Can you work these out from the model? Positions are in its coordinate system, mm. Coordinates: 2 decimals unless noted, no trailing zeros. Loops run counter-clockwise (first coordinate to the right, second up) from the corner with the lowest first, then second, coordinate; pieces in that order, holes last.
```python
from build123d import *

# Parameters (mm, degrees)
SKETCH1_R           = 88.9
BOSS_EXTRUDE1_DEPTH = 3.175
CUT_EXTRUDE3_DEPTH  = 1.5875
SKETCH3_R           = 14.224
CUT_EXTRUDE4_DEPTH  = 4.175
CUT_EXTRUDE5_DEPTH  = 4.175


with BuildPart() as part:
    # Sketch1 → Boss-Extrude1 (new body)
    with BuildSketch(Plane.XY):
        Circle(SKETCH1_R)
    extrude(amount=BOSS_EXTRUDE1_DEPTH)

    # Sketch2 → Cut-Extrude3 (cut)
    with BuildSketch(Plane(origin=(0, 0, 0), x_dir=(-1, 0, 0), z_dir=(0, 0, -1))):
        with BuildLine():
            ThreePointArc((-77.771132281, -43.068097053), (-76.989658396, -44.45), (-76.183632281, -45.81772771))
            Line((-76.183632281, -45.81772771), (-1.5875, -2.749630657))
            Line((-1.5875, -2.749630657), (-1.5875, -41.700369343))
            ThreePointArc((-1.5875, -41.700369343), (0, -41.275), (1.5875, -41.700369343))
            Line((1.5875, -41.700369343), (1.5875, -2.749630657))
            Line((1.5875, -2.749630657), (76.183632281, -45.81772771))
            ThreePointArc((76.183632281, -45.81772771), (76.989658396, -44.45), (77.771132281, -43.068097053))
            Line((77.771132281, -43.068097053), (3.175, 0))
            Line((3.175, 0), (36.907329198, 19.475369343))
            ThreePointArc((36.907329198, 19.475369343), (35.745198541, 20.6375), (35.319829198, 22.225))
            Line((35.319829198, 22.225), (1.5875, 2.749630657))
            Line((1.5875, 2.749630657), (1.5875, 88.885824763))
            ThreePointArc((1.5875, 88.885824763), (0, 88.9), (-1.5875, 88.885824763))
            Line((-1.5875, 88.885824763), (-1.5875, 2.749630657))
            Line((-1.5875, 2.749630657), (-35.319829198, 22.225))
            ThreePointArc((-35.319829198, 22.225), (-35.745198541, 20.6375), (-36.907329198, 19.475369343))
            Line((-36.907329198, 19.475369343), (-3.175, 0))
            Line((-3.175, 0), (-77.771132281, -43.068097053))
        make_face()
    extrude(amount=-CUT_EXTRUDE3_DEPTH, mode=Mode.SUBTRACT)

    # Sketch3 → Cut-Extrude4 (cut, through all)
    with BuildSketch(Plane.XY.offset(3.175)):
        Circle(SKETCH3_R)
    extrude(amount=-CUT_EXTRUDE4_DEPTH, mode=Mode.SUBTRACT)

    # Sketch2_4 → Cut-Extrude5 (cut, through all)
    with BuildSketch(Plane(origin=(0, 0, 0), x_dir=(-1, 0, 0), z_dir=(0, 0, -1))):
        with BuildLine():
            Line((-41.669829198, 22.225), (-36.907329198, 19.475369343))
            ThreePointArc((-36.907329198, 19.475369343), (-35.745198541, 20.6375), (-35.319829198, 22.225))
            Line((-35.319829198, 22.225), (-40.082329198, 24.974630657))
            ThreePointArc((-40.082329198, 24.974630657), (-41.244459855, 23.8125), (-41.669829198, 22.225))
        make_face()
        with BuildLine():
            ThreePointArc((-41.669829198, 22.225), (-40.082329198, 19.475369343), (-36.907329198, 19.475369343))
            Line((-36.907329198, 19.475369343), (-41.669829198, 22.225))
        make_face()
        with BuildLine():
            Line((-40.082329198, 24.974630657), (-35.319829198, 22.225))
            ThreePointArc((-35.319829198, 22.225), (-36.907329198, 24.974630657), (-40.082329198, 24.974630657))
        make_face()
        with BuildLine():
            ThreePointArc((35.319829198, 22.225), (35.745198541, 20.6375), (36.907329198, 19.475369343))
            Line((36.907329198, 19.475369343), (41.669829198, 22.225))
            ThreePointArc((41.669829198, 22.225), (41.244459855, 23.8125), (40.082329198, 24.974630657))
            Line((40.082329198, 24.974630657), (35.319829198, 22.225))
        make_face()
        with BuildLine():
            ThreePointArc((40.082329198, 24.974630657), (36.907329198, 24.974630657), (35.319829198, 22.225))
            Line((35.319829198, 22.225), (40.082329198, 24.974630657))
        make_face()
        with BuildLine():
            Line((41.669829198, 22.225), (36.907329198, 19.475369343))
            ThreePointArc((36.907329198, 19.475369343), (40.082329198, 19.475369343), (41.669829198, 22.225))
        make_face()
        with BuildLine():
            Line((-1.5875, -47.199630657), (-1.5875, -41.700369343))
            ThreePointArc((-1.5875, -41.700369343), (-3.175, -44.45), (-1.5875, -47.199630657))
        make_face()
        with BuildLine():
            ThreePointArc((1.5875, -41.700369343), (0, -41.275), (-1.5875, -41.700369343))
            Line((-1.5875, -41.700369343), (-1.5875, -47.199630657))
            ThreePointArc((-1.5875, -47.199630657), (0, -47.625), (1.5875, -47.199630657))
            Line((1.5875, -47.199630657), (1.5875, -41.700369343))
        make_face()
        with BuildLine():
            ThreePointArc((3.175, -44.45), (2.749630657, -42.8625), (1.5875, -41.700369343))
            Line((1.5875, -41.700369343), (1.5875, -47.199630657))
            ThreePointArc((1.5875, -47.199630657), (2.749630657, -46.0375), (3.175, -44.45))
        make_face()
    extrude(amount=-CUT_EXTRUDE5_DEPTH, mode=Mode.SUBTRACT)


solid = part.part
```
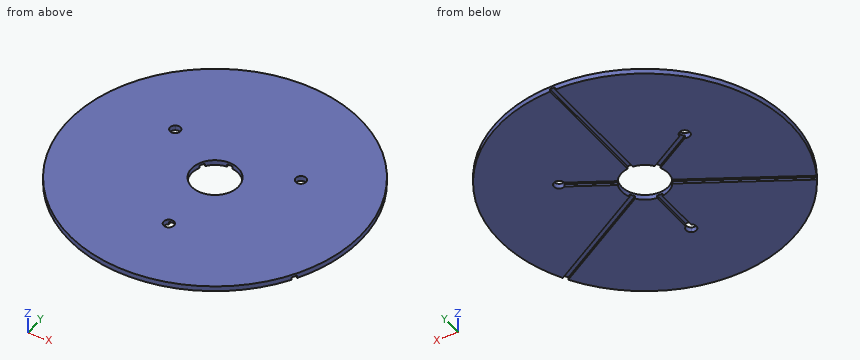
Item 1: Suppose I cut it at A-A, the plane z = 0.85. Count the separate pieces of the cut face and the enclosed holes in it, plus the area to 3 significant figures.
Results are:
separate pieces: 3
enclosed holes: 0
area: 23,100 mm2
Item 2: I need wall thicknesses on line 1 along X through (y, z) = (23.5, 3); line 2 along X through (y, z) = (37, 1.5); line 3 along Y through (x, z) = (0, 1.25) (3 decimals). Which ranges of each line are inside material? Lowest first, please.
Results are:
line 1: x = -85.74 to -41.4, -35.59 to 35.59, 41.4 to 85.74
line 2: x = -80.83 to -1.59, 1.59 to 80.83
line 3: y = -88.9 to -47.625
Item 3: Suppose I cut it at D-D, the plane x = -61. Please give me the cut outline in (y, z) (1 decimal).
Results are:
outline: (-64.7, 0) - (-37.1, 0) - (-37.1, 1.6) - (-33.4, 1.6) - (-33.4, 0) - (64.7, 0) - (64.7, 3.2) - (-64.7, 3.2) - close
Item 4: Suppose I cut it at C-C, the plane x = -8. Please give me the cut outline in (y, z) (3 decimals).
Results are:
outline: (-88.539, 0) - (-11.761, 0) - (-11.761, 3.175) - (-88.539, 3.175) - close; (11.761, 0) - (88.539, 0) - (88.539, 3.175) - (11.761, 3.175) - close
Item 5: Suppose I cut it at B-B, the plane y = 0. Please give me the cut outline in (x, z) (3 decimals), plus the area to 3 significant figures.
Results are:
outline: (-88.9, 0) - (-14.224, 0) - (-14.224, 3.175) - (-88.9, 3.175) - close; (14.224, 0) - (88.9, 0) - (88.9, 3.175) - (14.224, 3.175) - close
area: 474 mm2
Item 6: I'm going to push flat-ended pins straight in: P1, Ø1, axis at y = 9, z = 2.5, coming from the +X side; P2, Ø1.7, axis at y = 37, z = 1, coming from the +X side; P3, Ø1.3, axis at y = -33, z = 0.5, coming from the -X side. Where does each tip first touch, or does it pass through?
Results are:
P1: stops at x = 88.49
P2: stops at x = 81.22
P3: stops at x = -82.81
